The model under review builds one solid part; all positions refer to its coordinate system, in mm. A direction names the side the tool comes from. Coordinates: 2 decimals unless noted, no trailing zeros. Write each loop counter-clockwise with the first axis right and the second up, starting at its lowest first coordinate (ties: lowest second). Pieces come first, ordered by that corner, then holes.
```python
from build123d import *

# Parameters (mm, degrees)
SKETCH1_R           = 25
SKETCH1_R_2         = 16
BOSS_EXTRUDE1_DEPTH = 26.5
SKETCH1_3_R         = 16
BOSS_EXTRUDE2_DEPTH = 5
SKETCH2_R           = 2
CUT_EXTRUDE1_DEPTH  = 5
SKETCH3_R           = 2.55
CUT_EXTRUDE2_DEPTH  = 5
SKETCH5_R           = 7.5
CUT_EXTRUDE8_DEPTH  = 19
SKETCH6_W           = 8
SKETCH6_H           = 5
CUT_EXTRUDE9_DEPTH  = 19


with BuildPart() as part:
    # Sketch1 → Boss-Extrude1 (new body)
    # profile 1 of 4: a face of its own
    with BuildSketch(Plane(origin=(0, 0, 0), x_dir=(1, 0, 0), z_dir=(0, 1, 0))):
        Circle(SKETCH1_R)
        with Locations(Location((0, 0, 0), (0, 0, 270))):
            Circle(SKETCH1_R_2, mode=Mode.SUBTRACT)
    # profile 2 of 4: a face of its own
    with BuildSketch(Plane(origin=(0, 0, 0), x_dir=(1, 0, 0), z_dir=(0, 1, 0))):
        with BuildLine():
            ThreePointArc((0, -25), (-17.67766953, -17.67766953), (-25, 0))
            Line((-25, 0), (-25, -25))
            Line((-25, -25), (0, -25))
        make_face()
    # profile 3 of 4: a face of its own
    with BuildSketch(Plane(origin=(0, 0, 0), x_dir=(1, 0, 0), z_dir=(0, 1, 0))):
        with BuildLine():
            ThreePointArc((-25, 0), (-17.67766953, 17.67766953), (0, 25))
            Line((0, 25), (-25, 25))
            Line((-25, 25), (-25, 0))
        make_face()
    # profile 4 of 4: a face of its own
    with BuildSketch(Plane(origin=(0, 0, 0), x_dir=(1, 0, 0), z_dir=(0, 1, 0))):
        with BuildLine():
            Line((25, 25), (0, 25))
            ThreePointArc((0, 25), (17.67766953, 17.67766953), (25, 0))
            Line((25, 0), (25, 25))
        make_face()
    extrude(amount=BOSS_EXTRUDE1_DEPTH)

    # Sketch1_3 → Boss-Extrude2 (add)
    with BuildSketch(Plane(origin=(0, 0, 0), x_dir=(1, 0, 0), z_dir=(0, 1, 0))):
        with Locations(Location((0, 0, 0), (0, 0, 270))):
            Circle(SKETCH1_3_R)
    extrude(amount=BOSS_EXTRUDE2_DEPTH)

    # Sketch2 → Cut-Extrude1 (cut)
    with BuildSketch(Plane(origin=(0, 5, 0), x_dir=(1, 0, 0), z_dir=(0, 1, 0))):
        with Locations(Location((0, 0, 0), (0, 0, 270))):
            Circle(SKETCH2_R)
    extrude(amount=-CUT_EXTRUDE1_DEPTH, mode=Mode.SUBTRACT)

    # Sketch3 → Cut-Extrude2 (cut)
    with BuildSketch(Plane.ZY.offset(25)):
        with Locations((0, 15)):
            Circle(SKETCH3_R)
    extrude(amount=-CUT_EXTRUDE2_DEPTH, mode=Mode.SUBTRACT)

    # Sketch5 → Cut-Extrude8 (cut)
    with BuildSketch(Plane.XY):
        with Locations((0, 12.5)):
            Circle(SKETCH5_R)
    extrude(amount=-CUT_EXTRUDE8_DEPTH, mode=Mode.SUBTRACT)

    # Sketch6 → Cut-Extrude9 (cut)
    with BuildSketch(Plane.XY.offset(-19)):
        with Locations((0, 12.5)):
            Rectangle(SKETCH6_W, SKETCH6_H)
    extrude(amount=-CUT_EXTRUDE9_DEPTH, mode=Mode.SUBTRACT)


solid = part.part
```
Item 1: Machinability: for faces 4 (the face through (-6.13, 15.6, 14.78)), 5 (the face through (4, 12, -22)), 6 (the face through (0, 9, -19)), which of the approach directions +Z, -Z, +X, -X, +Y, -Y give a long, thin tool a straight path to every point of the face, cutting with its end or side? Answer none if there is none.
Solved:
face 4: +Y
face 5: -Z
face 6: none
Item 2: Take a section at D-D, the plane y = 11. Write out the cut boundary in (x, z).
Solved:
outline: (-25, -25) - (-4, -25) - (-4, -19) - (-7.35, -19) - (-7.35, -14.21) arc R16 cw (long way) to (7.35, -14.21) - (7.35, -19) - (4, -19) - (4, -25) - (25, -25) - (25, 0) arc R25 ccw to (0, 25) - (-25, 25) - close
Item 3: To check wall thickness, follow line 1 along Z through (x, y) = (0, 21.75); line 2 along X through (y, z) = (12.5, -16.3); line 3 along Y through (x, z) = (-22.2, 0). State the ranges of each line that lie inside material, in increasing order.
Solved:
line 1: z = -25 to -16, 16 to 25
line 2: x = -25 to -7.5, 7.5 to 25
line 3: y = 0 to 12.45, 17.55 to 26.5
Item 4: For pin 1 (3 mm diameter, centred on y = 15, z = 0, fed in from -X), flat-tipped, find the tip position at first contact; note if it passes through.
Solved:
pin 1: stops at x = -20
Item 5: Take a section at C-C, the plane z = -7. Write out the cut boundary in (x, y).
Solved:
outline: (-25, 0) - (25, 0) - (25, 26.5) - (14.39, 26.5) - (14.39, 5) - (-14.39, 5) - (-14.39, 26.5) - (-25, 26.5) - close
Item 6: Take a section at B-B, the plane x = 10. Write out the cut boundary in (y, z), plus the area to 3 significant figures.
Solved:
outline: (0, -25) - (26.5, -25) - (26.5, -12.49) - (5, -12.49) - (5, 12.49) - (26.5, 12.49) - (26.5, 22.91) - (0, 22.91) - close
area: 733 mm2
Item 7: Mouldability with a two-part tool opening along Y and no side actions: class faces 1 (the face through (-6, 8, -17)), 2 (the face through (17.482, 13.064, 17.871)), 3 (the face through (-11.5, 26.5, -11.5)) as pulls with the +Y half, pulls with the -Y half, needs draft (parallel to the pull), parting line crosses it, or undercut.
Solved:
face 1: undercut
face 2: needs draft
face 3: pulls with the +Y half
Item 8: Take a section at A-A, the plane z = -17.5. Write out the cut boundary in (x, y), plus the area to 3 significant figures.
Solved:
outline: (-25, 0) - (25, 0) - (25, 26.5) - (-25, 26.5) - close; hole circle Ø15 at (0, 12.5)
area: 1,150 mm2
